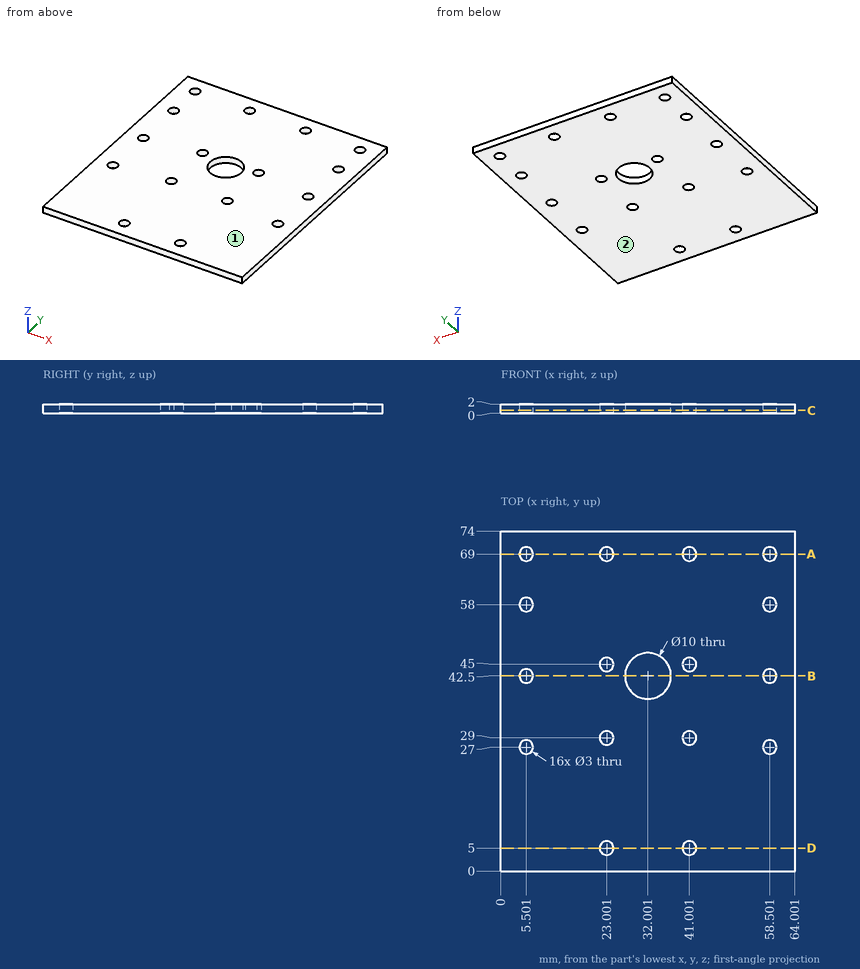
Drawing for the job (mm, zero at the part's lowest x, y, z). Round coordinates to 2 decimals unless told otherwise and drop trailing zeros. Loops run counter-clockwise (first coordinate to the right, second up) from the corner with the lowest first, then second, coordinate; pieces in that order, holes last. Notation, with made-up numbers: (-15.75, 27) -> (21.25, 27) arc R10 cw to (21.25, 36) -> close; hole circle Ø2 at (22.25, 50). An arc over 180 degrees is marked (long way). Use one line per item in the form item = value. Start each with the question number.
Item 1: Drop flat-ended pins along their axis: pin 1 Ø5 at (x, y) = (41, 69) entering from +Z; pin 2 Ø8 at (x, y) = (32, 42.5) entering from +Z. Give the stop position or say it passes through.
Item 2: Drill centre lines: line 1 along Y through (x, z) = (5.5, 0.35); line 2 along Y through (x, z) = (40.5, 1.35) (1 decimal); line 3 along Y through (x, z) = (30, 1.35). Where is each one in solid material? Low to high.
Item 3: Band-saw the part on B-B (y = 42.5). List the corners of the cut face in (x, z).
Item 4: Band-saw the part on C-C (z = 0.6). Give the number of separate pieces and of enclosed holes in the cut face, plus the area to 3 significant figures.
Item 5: Band-saw the part on A-A (y = 69). List the corners of the cut face in (x, z).
Item 6: Two-plate mould, pull along Z, no slides. Class the marked faces 1 and 2: released by +Z, released by -Z, zero draft, split by the parting line, or undercut.
Item 7: Band-saw the part on D-D (y = 5). List the corners of the cut face in (x, z), plus the area to 3 significant figures.
Data:
q1.pin_1 = 2
q1.pin_2 = through
q2.line_1 = 0 to 25.5, 28.5 to 41, 44 to 56.5, 59.5 to 67.5, 70.5 to 74
q2.line_2 = 0 to 3.6, 6.4 to 27.6, 30.4 to 43.6, 46.4 to 67.6, 70.4 to 74
q2.line_3 = 0 to 37.92, 47.08 to 74
q3.outline = (0, 0) -> (4, 0) -> (4, 2) -> (0, 2) -> close; (7, 0) -> (27, 0) -> (27, 2) -> (7, 2) -> close; (37, 0) -> (57, 0) -> (57, 2) -> (37, 2) -> close; (60, 0) -> (64, 0) -> (64, 2) -> (60, 2) -> close
q4.separate_pieces = 1
q4.enclosed_holes = 17
q4.area = 4,540 mm^2
q5.outline = (0, 0) -> (4, 0) -> (4, 2) -> (0, 2) -> close; (7, 0) -> (21.5, 0) -> (21.5, 2) -> (7, 2) -> close; (24.5, 0) -> (39.5, 0) -> (39.5, 2) -> (24.5, 2) -> close; (42.5, 0) -> (57, 0) -> (57, 2) -> (42.5, 2) -> close; (60, 0) -> (64, 0) -> (64, 2) -> (60, 2) -> close
q6.face_1 = released by +Z
q6.face_2 = released by -Z
q7.outline = (0, 0) -> (21.5, 0) -> (21.5, 2) -> (0, 2) -> close; (24.5, 0) -> (39.5, 0) -> (39.5, 2) -> (24.5, 2) -> close; (42.5, 0) -> (64, 0) -> (64, 2) -> (42.5, 2) -> close
q7.area = 116 mm^2
